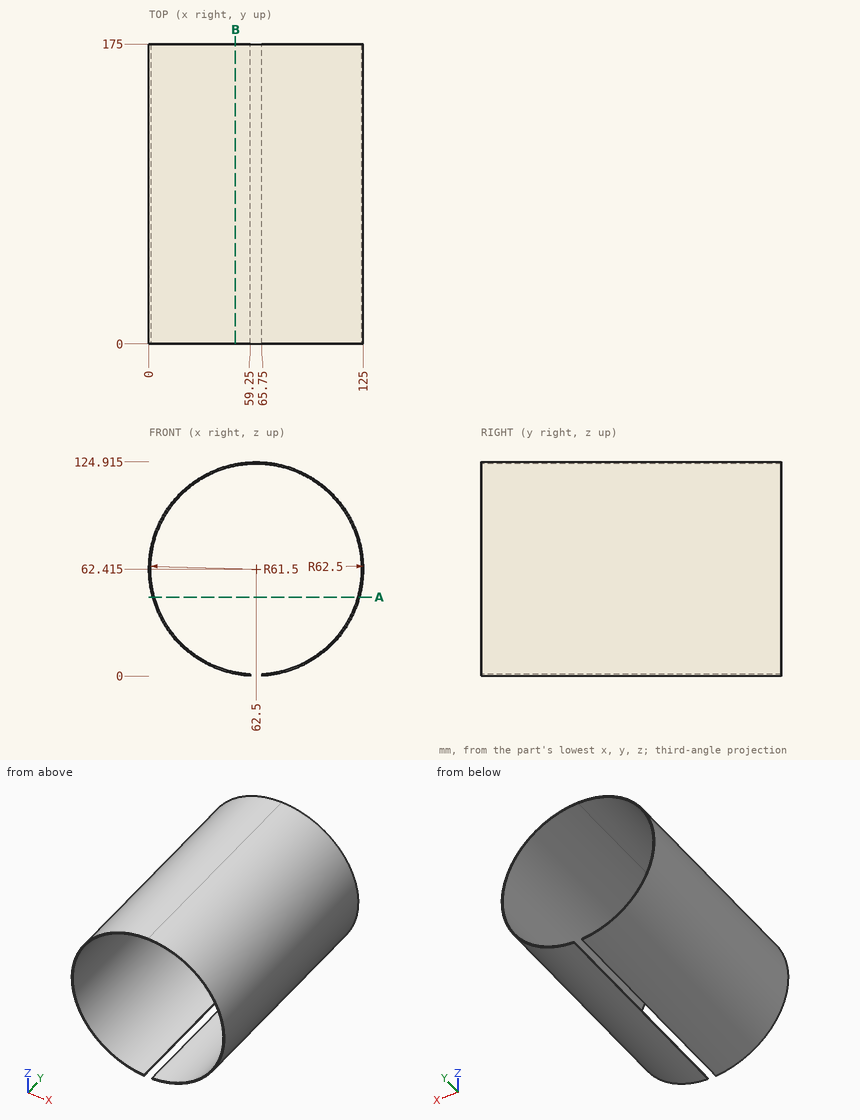
Can you work these out from the drawing? Everything is in mm from the part's minimum corner. Give positions to 0.01 mm unless a question says otherwise; leave off trailing zeros. Order: outer loops, then holes, each group sorted by start corner. A loop starts at its lowest first (then second) coordinate and runs counter-clockwise, first axis right, second up.
Item 1: If we section it at A-A, the plane z = 46: Write out the boundary of the cut face in (x, y) (1 decimal).
Item 2: If we section it at B-B, the plane x = 50.5: Write out the boundary of the cut face in (y, z).
Item 3: I'm going to push flat-ended pins straight in: pin 1 (1 mm diameter, centred on x = 50.5, y = 48, fed in from +Z); pin 2 (5 mm diameter, centred on y = 47.5, z = 40, fed in from -X); pin 3 (5 mm diameter, centred on x = 25, y = 102, fed in from -Z) (1 decimal). Where does each tip first touch, or does it pass through?
Item 4: I need wall thicknesses on line 1 (X direction, y = 66.5, z = 94.5) (1 decimal); line 2 (Z direction, x = 71.5, y = 16) (1 decimal); line 3 (Z direction, x = 57, y = 96). Which ranges of each line are inside material? Lowest first, please.
Values:
1. outline: (2.2, 0) - (3.2, 0) - (3.2, 175) - (2.2, 175) - close; (121.8, 0) - (122.8, 0) - (122.8, 175) - (121.8, 175) - close
2. outline: (0, 1.08) - (175, 1.08) - (175, 2.1) - (0, 2.1) - close; (0, 122.73) - (175, 122.73) - (175, 123.75) - (0, 123.75) - close
3. pin 1: stops at z = 123.85
3. pin 2: stops at x = 3.26
3. pin 3: stops at z = 10.6
4. line 1: x = 8.9 to 10, 115 to 116.1
4. line 2: z = 0.6 to 1.6, 123.3 to 124.3
4. line 3: z = 0.16 to 1.16, 123.67 to 124.67
